```python
from build123d import *

# Parameters (mm, degrees)
BOSS_EXTRUDE1_DEPTH = 5
SKETCH2_W           = 113
SKETCH2_H           = 35
SKETCH2_H_2         = 12.5
CUT_EXTRUDE1_DEPTH  = 10


with BuildPart() as part:
    # Sketch1 → Boss-Extrude1 (new body)
    with BuildSketch(Plane(origin=(0, 0, 0), x_dir=(1, 0, 0), z_dir=(0, 1, 0))):
        Polygon((-80, 71.5), (-80, 51.5), (-75, 51.5), (-75, 30.5), (-80, 30.5), (-80, 10.5), (-75, 10.5), (-75, -10.5), (-80, -10.5), (-80, -30.5), (-75, -30.5), (-75, -51.5), (-80, -51.5), (-80, -71.5), (-75, -71.5), (-75, -92.5), (-80, -92.5), (-80, -112.5), (-75, -112.5), (-75, -132.5), (-70, -132.5), (-70, -127.5), (-54.25, -127.5), (-54.25, -132.5), (-38.9375, -132.5), (-38.9375, -127.5), (-23.1875, -127.5), (-23.1875, -132.5), (-7.875, -132.5), (-7.875, -127.5), (7.875, -127.5), (7.875, -132.5), (23.1875, -132.5), (23.1875, -127.5), (38.9375, -127.5), (38.9375, -132.5), (54.25, -132.5), (54.25, -127.5), (70, -127.5), (70, -132.5), (75, -132.5), (75, -112.5), (80, -112.5), (80, -92.5), (75, -92.5), (75, -71.5), (80, -71.5), (80, -51.5), (75, -51.5), (75, -30.5), (80, -30.5), (80, -10.5), (75, -10.5), (75, 10.5), (80, 10.5), (80, 30.5), (75, 30.5), (75, 51.5), (80, 51.5), (80, 71.5), (75, 71.5), (75, 92.5), (80, 92.5), (80, 112.5), (75, 112.5), (75, 132.5), (70, 132.5), (70, 127.5), (54.25, 127.5), (54.25, 132.5), (38.9375, 132.5), (38.9375, 127.5), (23.1875, 127.5), (23.1875, 132.5), (7.875, 132.5), (7.875, 127.5), (-7.875, 127.5), (-7.875, 132.5), (-23.1875, 132.5), (-23.1875, 127.5), (-38.9375, 127.5), (-38.9375, 132.5), (-54.25, 132.5), (-54.25, 127.5), (-70, 127.5), (-70, 132.5), (-75, 132.5), (-75, 112.5), (-80, 112.5), (-80, 92.5), (-75, 92.5), (-75, 71.5), align=None)
    extrude(amount=BOSS_EXTRUDE1_DEPTH)

    # Sketch2 → Cut-Extrude1 (cut)
    with BuildSketch(Plane(origin=(0, 5, 0), x_dir=(1, 0, 0), z_dir=(0, 1, 0))):
        with Locations((0, 2)):
            Rectangle(SKETCH2_W, SKETCH2_H)
        with Locations((0, -36.75)):
            Rectangle(SKETCH2_W, SKETCH2_H_2)
    extrude(amount=-CUT_EXTRUDE1_DEPTH, mode=Mode.SUBTRACT)


solid = part.part
```
Can you work these out from the model? Positions are in its coordinate system, mm. A direction names the side the tool comes from. Give positions to 0.01 mm unless a question says otherwise; leave off trailing zeros. Loops run counter-clockwise (first coordinate to the right, second up) from the corner with the lowest first, then second, coordinate; pieces in that order, holes last. Notation, with made-up numbers: M 50.25,57.5 L 88.25,57.5 A19 cw 88.25,68.5 Z; hole C 16,64.25 d6. An arc over 180 degrees is marked long. Use CSV: the item, a comma, the result in double quotes. Start each with the question number.
1. Imagine slicing it at C-C, the plane x = -49. Write out the boundary of the cut face in (y, z), plus the area to 3 significant figures.
2. Imagine slicing it at A-A, the plane x = 33. Write out the boundary of the cut face in (y, z).
3. Imagine slicing it at D-D, the plane z = -79. Write out the boundary of the cut face in (x, y), plus the area to 3 significant figures.
4. If we mould it in two halves opening along X, with no side actions, what happens to faces 6 (the face through (-7.875, 2, -130)), 7 (the face through (-75, 2, -82)), 8 (the face through (78, 2, 92.5)), 9 (the face through (-1, 3, 15.5))? For each: released by +X, released by -X, zero draft, split by the parting line, or undercut.
5. For P1, Ø2.5, axis at y = 2.5, z = 129.5, coming from the +X side; P2, Ø2, axis at x = -11.5, z = 86.5, coming from the -Y side; P3, Ø2.5, axis at y = 3.5, z = 81.5, coming from the -X side; P4, Ø1.5, axis at x = 76.5, y = 1.5, coming from the -Z side, each with a flat end and sliding along its axis, tell me the tip position at first contact or that it passes through.
6. If I drill on L1, parallel to Z at x = 45, y = 0.55; L2, parallel to Z at x = -37.5, y = 0.8; L3, parallel to X at y = 2.3, z = 40, over which ranges is the centre line in solid material (lowest first)?
7. Imagine slicing it at B-B, the plane y = 3. Count the separate pieces of the cut face and the enclosed holes in it, plus the area to 3 significant figures.
8. On a 3-axis mill with a long thin cutter (end or side, diameter ignored), from which of +Z, -Z, +X, -X, +Y, -Y can I reach the whole of each face in a straight line? I mean faces 1 (the face through (-31, 2, -127.5)), 2 (the face through (-78, 2, -51.5)), 3 (the face through (75, 2, -41)), 4 (the face through (-62, 2, 127.5)), 5 (the face through (-80, 2, -21)). Say none if no direction works.
Response values:
1,outline,"M 0,-132.5 L 5,-132.5 L 5,-19.5 L 0,-19.5 Z; M 0,15.5 L 5,15.5 L 5,30.5 L 0,30.5 Z; M 0,43 L 5,43 L 5,132.5 L 0,132.5 Z"
1,area,"1,090 mm^2"
2,outline,"M 0,-127.5 L 5,-127.5 L 5,-19.5 L 0,-19.5 Z; M 0,15.5 L 5,15.5 L 5,30.5 L 0,30.5 Z; M 0,43 L 5,43 L 5,127.5 L 0,127.5 Z"
3,outline,"M -75,0 L 75,0 L 75,5 L -75,5 Z"
3,area,"750 mm^2"
4,face 6,"undercut"
4,face 7,"released by -X"
4,face 8,"zero draft"
4,face 9,"undercut"
5,P1,"x = 75"
5,P2,"y = 0"
5,P3,"x = -75"
5,P4,"z = -112.5"
6,L1,"-132.5 to -19.5, 15.5 to 30.5, 43 to 132.5"
6,L2,"-127.5 to -19.5, 15.5 to 30.5, 43 to 127.5"
6,L3,"-75 to -56.5, 56.5 to 75"
7,separate pieces,"1"
7,enclosed holes,"2"
7,area,"34,800 mm^2"
8,face 1,"-Z, +Y, -Y"
8,face 2,"-X, +Y, -Y"
8,face 3,"+X, +Y, -Y"
8,face 4,"+Z, +Y, -Y"
8,face 5,"+Z, -Z, -X, +Y, -Y"
